```python
from build123d import *

# Parameters (mm, degrees)
SKETCH1_W           = 14
SKETCH1_H           = 14
BOSS_EXTRUDE1_DEPTH = 1.6
SKETCH2_R           = 7
SKETCH2_R_2         = 6
BOSS_EXTRUDE2_DEPTH = 1.6
SKETCH3_R           = 6
CUT_EXTRUDE1_DEPTH  = 2.6


with BuildPart() as part:
    # Sketch1 → Boss-Extrude1 (new body)
    with BuildSketch(Plane(origin=(0, 0, 0), x_dir=(1, 0, 0), z_dir=(0, 1, 0))):
        Rectangle(SKETCH1_W, SKETCH1_H)
    extrude(amount=BOSS_EXTRUDE1_DEPTH)

    # Sketch2 → Boss-Extrude2 (add)
    with BuildSketch(Plane(origin=(0, 1.6, 0), x_dir=(1, 0, 0), z_dir=(0, 1, 0))):
        Circle(SKETCH2_R)
        Circle(SKETCH2_R_2, mode=Mode.SUBTRACT)
    extrude(amount=BOSS_EXTRUDE2_DEPTH)

    # Sketch3 → Cut-Extrude1 (cut, through all)
    with BuildSketch(Plane(origin=(0, 1.6, 0), x_dir=(1, 0, 0), z_dir=(0, 1, 0))):
        Circle(SKETCH3_R)
    extrude(amount=-CUT_EXTRUDE1_DEPTH, mode=Mode.SUBTRACT)


solid = part.part
```
Here's how the part is built. I have some questions about the finished solid (model axes, mm). A direction names the side the tool comes from. Round coordinates to 2 decimals unless told otherwise and drop trailing zeros. Order: outer loops, then holes, each group sorted by start corner. A loop starts at its lowest first (then second) coordinate and runs counter-clockwise, first axis right, second up. Notation, with made-up numbers: M -26.75,66.5 L -3.75,66.5 A22 cw -3.75,96.5 Z; hole C 79.25,-12 d10. An arc over 180 degrees is marked long. Answer in a Markdown table with one row per item.
Item 1: For faces 1 (the face through (6, 1.6, 6)), 2 (the face through (5, 1.6, -6)), 3 (the face through (-6, 1.6, 5)), which set-ups out of +Z, -Z, +X, -X, +Y, -Y let a thin tool reach every point of the face, with its end or its side?
A:
| item | result |
|---|---|
| face 1 | +Z, +X, +Y |
| face 2 | -Z, +X, +Y |
| face 3 | +Z, -X, +Y |
Item 2: Imagine slicing it at B-B, the plane z = -3.25. Write out the boundary of the cut face in (x, y).
A:
| item | result |
|---|---|
| outline | M -7,0 L -5.04,0 L -5.04,3.2 L -6.2,3.2 L -6.2,1.6 L -7,1.6 Z; M 5.04,0 L 7,0 L 7,1.6 L 6.2,1.6 L 6.2,3.2 L 5.04,3.2 Z |
Item 3: If I drill on L1, parallel to Z at x = 0, y = 1.1; L2, parallel to Z at x = 5.5, y = 3.05, over which ranges is the centre line in solid material (lowest first)? Write a range as from..to.
A:
| item | result |
|---|---|
| L1 | z = -7..-6, 6..7 |
| L2 | z = -4.33..-2.4, 2.4..4.33 |
Item 4: Imagine slicing it at D-D, the plane y = 1.85. Write out the boundary of the cut face in (x, z).
A:
| item | result |
|---|---|
| outline | C 0,0 d14; hole C 0,0 d12 |
Item 5: Imagine slicing it at C-C, the plane y = 0.7. Write out the boundary of the cut face in (x, z).
A:
| item | result |
|---|---|
| outline | M -7,-7 L 7,-7 L 7,7 L -7,7 Z; hole C 0,0 d12 |
Item 6: I'm going to push a flat-ended pin straight in: pin 1 (1.5 mm diameter, centred on x = 1, y = 2.5, fed in from -Z). Where does the tip first touch, or does it pass through?
A:
| item | result |
|---|---|
| pin 1 | stops at z = -7 |
Item 7: Imagine slicing it at A-A, the plane x = -3.75. Write out the boundary of the cut face in (y, z).
A:
| item | result |
|---|---|
| outline | M 0,-7 L 1.6,-7 L 1.6,-5.91 L 3.2,-5.91 L 3.2,-4.68 L 0,-4.68 Z; M 0,4.68 L 3.2,4.68 L 3.2,5.91 L 1.6,5.91 L 1.6,7 L 0,7 Z |
